Answer from the drawing. Dimensions are ordinates in mm from the lowest x, y and z of the part. Round coordinates to 2 decimals unless told otherwise and drop trailing zeros. Order: outer loops, then holes, each group sorted by start corner. A loop starts at its lowest first (then second) coordinate and runs counter-clockwise, first axis right, second up. Notation, with made-up numbers: M 25,11 L 32,11 A29 ccw 32,36 Z; hole C 27,54 d11. An arc over 180 degrees is marked long. Write item = value, one per line. Start each with the question number.
(1) For a pull along X with two mould halves and no side action, classify the marked faces 1 and 2 as released by +X, released by -X, zero draft, split by the parting line, or undercut.
(2) Straight lines are drawn through the part: probe 1 along X at (y, z) = (2.8, 66); probe 2 along X at (y, z) = (3.95, 15); probe 3 along Z at (x, y) = (73, 3.9). For each, find the intervals that lie inside material, in ascending order. Write a range as from..to.
(3) A cutting plane is placed at D-D, the plane z = 15. Determine the outline of the cut face in (x, y).
(4) A cutting plane is placed at B-B, the plane x = 73. Determine the outline of the cut face in (y, z).
(5) A cutting plane is placed at A-A, the plane z = 72. Determine the outline of the cut face in (x, y), and give its area (3 significant figures).
(6) Each of these flat-tipped pins is pushed along its axis until it touches: pin 1 (1.5 mm diameter, centred on x = 52.5, y = 6, fed in from +Z); pin 2 (4 mm diameter, centred on y = 3.5, z = 34, fed in from +X); pin 3 (1.8 mm diameter, centred on x = 67, z = 15, fed in from +Y). Where does it stop, or does it pass through?
(7) A cutting plane is placed at C-C, the plane x = 52.5. Determine the outline of the cut face in (y, z).
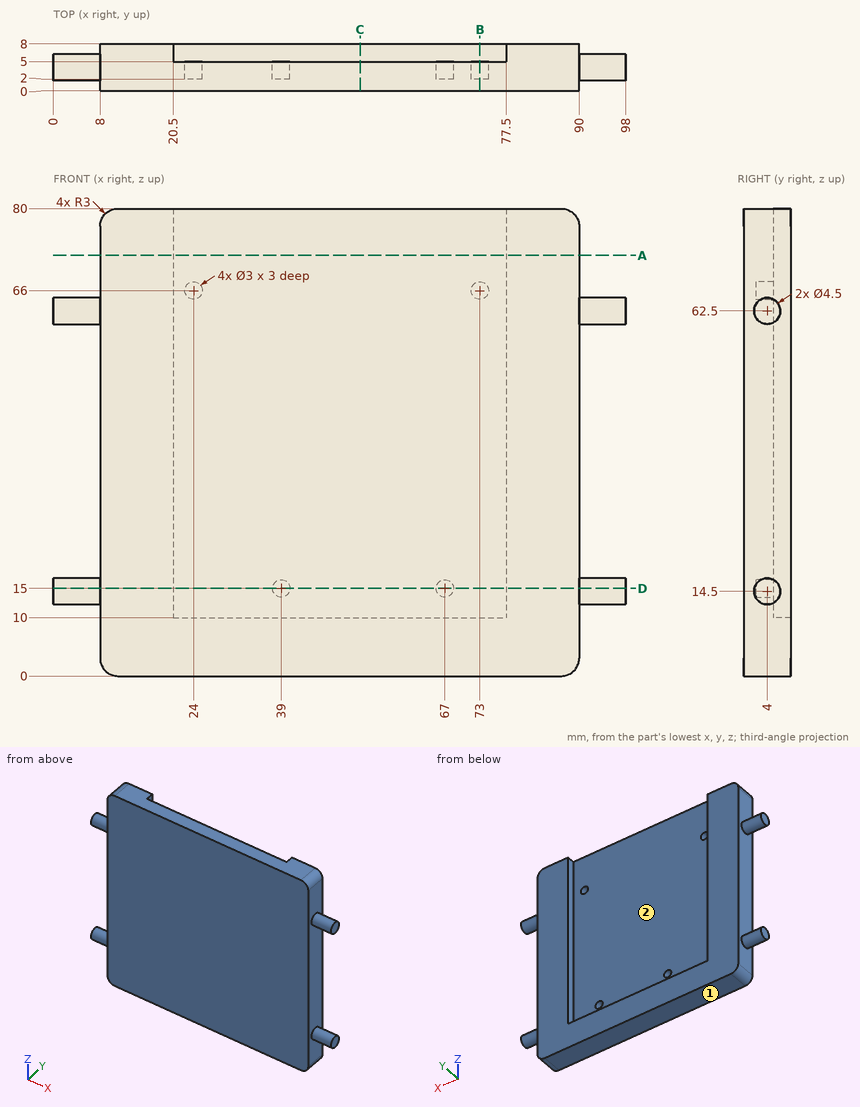
Reported:
q1.face_1 = zero draft
q1.face_2 = undercut
q2.probe_1 = 8..22.5, 25.5..71.5, 74.5..90
q2.probe_2 = 0..37.5, 40.5..65.5, 68.5..98
q2.probe_3 = 0..64.5, 67.5..80
q3.outline = M 0,1.81 L 8,1.81 L 8,0 L 90,0 L 90,1.81 L 98,1.81 L 98,6.19 L 90,6.19 L 90,8 L 77.5,8 L 77.5,5 L 68.5,5 L 68.5,2 L 65.5,2 L 65.5,5 L 40.5,5 L 40.5,2 L 37.5,2 L 37.5,5 L 20.5,5 L 20.5,8 L 8,8 L 8,6.19 L 0,6.19 Z
q4.outline = M 0,0 L 8,0 L 8,10 L 5,10 L 5,64.5 L 2,64.5 L 2,67.5 L 5,67.5 L 5,80 L 0,80 Z
q5.outline = M 8,0 L 90,0 L 90,8 L 77.5,8 L 77.5,5 L 20.5,5 L 20.5,8 L 8,8 Z
q5.area = 485 mm²
q6.pin_1 = 10
q6.pin_2 = 90
q6.pin_3 = 2
q7.outline = M 0,0 L 8,0 L 8,10 L 5,10 L 5,80 L 0,80 Z
